Autodesk Inventor part; units mm, degrees
ref_plane "YZ Plane" through (0, 0, 0) normal (1, 0, 0) x (0, 1, 0)
ref_plane "XZ Plane" through (0, 0, 0) normal (0, 1, 0) x (-1, 0, 0)
ref_plane "XY Plane" through (0, 0, 0) normal (0, 0, 1) x (1, 0, 0)
sketch "Skizze1" plane through (0, 0, 0) normal (0, 0, 1) x (1, 0, 0)
  line L0 (-5, -1.75) -> (5, -1.75)
  line L1 (5, -1.75) -> (5, 1.75)
  line L2 (5, 1.75) -> (-5, 1.75)
  line L3 (-5, 1.75) -> (-5, -1.75)
  line L4 (-5, -1.75) -> (5, 1.75) construction
  line L5 (5, -1.75) -> (-5, 1.75) construction
  line L6 (-9, -4.25) -> (9, -4.25)
  line L7 (9, -4.25) -> (9, 4.25)
  line L8 (9, 4.25) -> (-9, 4.25)
  line L9 (-9, 4.25) -> (-9, -4.25)
  line L10 (-9, -4.25) -> (9, 4.25) construction
  line L11 (9, -4.25) -> (-9, 4.25) construction
  line L12 (-9, -4.25) -> (-9, -7.25)
  line L13 (9, -4.25) -> (9, -7.25)
  arc A0 (9, -7.25) -> (-9, -7.25) centre (0, -19.25) ccw
  point P0 (0, 0)
  dimension "d0" = 10
  dimension "d1" = 3.5
  dimension "d2" = 18
  dimension "d3" = 2.5
  dimension "d4" = 3
extrude "Extrusion1" add sketch "Skizze1" along normal blind 13
sketch "Skizze2" plane through (0, 0, 0) normal (0, 0, -1) x (-1, 0, 0)
  line L0 (5, 1.75) -> (5, -1.75)
  line L1 (5, -1.75) -> (-5, -1.75)
  line L2 (-5, -1.75) -> (-5, 1.75)
  line L3 (-5, 1.75) -> (5, 1.75)
  line L4 (9, 4.25) -> (9, -7.25)
  line L5 (-9, 4.25) -> (9, 4.25)
  line L6 (-9, -7.25) -> (-9, 4.25)
  arc A0 (9, -7.25) -> (-9, -7.25) centre (0, -19.25) ccw
  point P0 (0, 0)
extrude "Extrusion2" add sketch "Skizze2" along normal blind 3 contours L0 L1 L2 L3 | L4 A0 L6 L5
fillet "Rundung1" radius 2 4 edges at (-5, 0, 13) (5, 0, 13) (0, 1.75, 13) (0, -1.75, 13)
properties part number "vibramount"
For this review, take the finished solid that the model builds, in its own axes (mm). A direction names the side the tool comes from. Give positions to 0.01 mm unless a question says otherwise; leave off trailing zeros. Loops run counter-clockwise (first coordinate to the right, second up) from the corner with the lowest first, then second, coordinate; pieces in that order, holes last. Notation, with made-up numbers: (5, -19.5) -> (29, -19.5) arc R13 cw to (29, 4.5) -> close; hole circle Ø2 at (42.25, -16.5). An arc over 180 degrees is marked (long way). One line per question, with ' | ' between items.
1) For faces 1 (the flat face through (0, -4, 13)), 2 (the flat face through (0, -1.75, 5)), list the 3-axis set-ups (+Z, -Z, +X, -X, +Y, -Y) from which the entire face can be reached by the end or side of a thin tool; tool diameter is ignored.
Resolved:
face 1: +Z, +X, -X, +Y, -Y | face 2: +Z
2) We need section A-A (z = 1.5). Write out the cut boundary in (x, y), plus the area to 3 significant figures.
Resolved:
outline: (-9, -7.25) arc R15 cw to (9, -7.25) -> (9, 4.25) -> (-9, 4.25) -> close; hole (-5, -1.75) -> (5, -1.75) -> (5, 1.75) -> (-5, 1.75) -> close | area: 135 mm2
3) We need section D-D (x = -6.25). Write out the cut boundary in (y, z), plus the area to 3 significant figures.
Resolved:
outline: (-5.61, -3) -> (4.25, -3) -> (4.25, 13) -> (3.75, 13) arc R2 ccw to (3, 12.85) -> (-3, 12.85) arc R2 ccw to (-3.75, 13) -> (-5.61, 13) -> close | area: 157 mm2
4) Insertion check: pin 1 Ø4 at (x, y) = (-0.5, 0.5) entering from +Z. The pin has a flat end and moves straight along its axis. Give the tip position at first contact, or say it passes through.
Resolved:
pin 1: stops at z = 12.56
5) The part is to be moulded in two halves that separate along X. For faces 3 (the flat face through (-9, -1, 5)), 4 (the flat face through (9, -2, 5)), 5 (the cylindrical face through (-0.14, -4.25, 4.89)), say which applies: +X half, -X half, draft (parallel to the pull), parting line (faces both ways), or undercut.
Resolved:
face 3: -X half | face 4: +X half | face 5: undercut
6) To check wall thickness, follow probe 1 along X at (y, z) = (1, 5.75); probe 2 along Y at (x, z) = (-3.25, 12); probe 3 along Y at (x, z) = (1.5, 7). State the ranges of each line that lie inside material, in increasing order.
Resolved:
probe 1: x = -9 to -5, 5 to 9 | probe 2: y = -4.61 to -2.02, 2.02 to 4.25 | probe 3: y = -4.33 to -1.75, 1.75 to 4.25
7) We need section B-B (y = 1). Write out the cut boundary in (x, z), plus the area to 3 significant figures.
Resolved:
outline: (-9, -3) -> (9, -3) -> (9, 13) -> (7, 13) arc R2 ccw to (5, 11) -> (5, 0) -> (-5, 0) -> (-5, 11) arc R2 ccw to (-7, 13) -> (-9, 13) -> close | area: 156 mm2
8) We need section C-C (y = -6.25). Write out the cut boundary in (x, z).
Resolved:
outline: (-9, -3) -> (-7.48, -3) -> (-7.48, 13) -> (-9, 13) -> close; (7.48, -3) -> (9, -3) -> (9, 13) -> (7.48, 13) -> close
